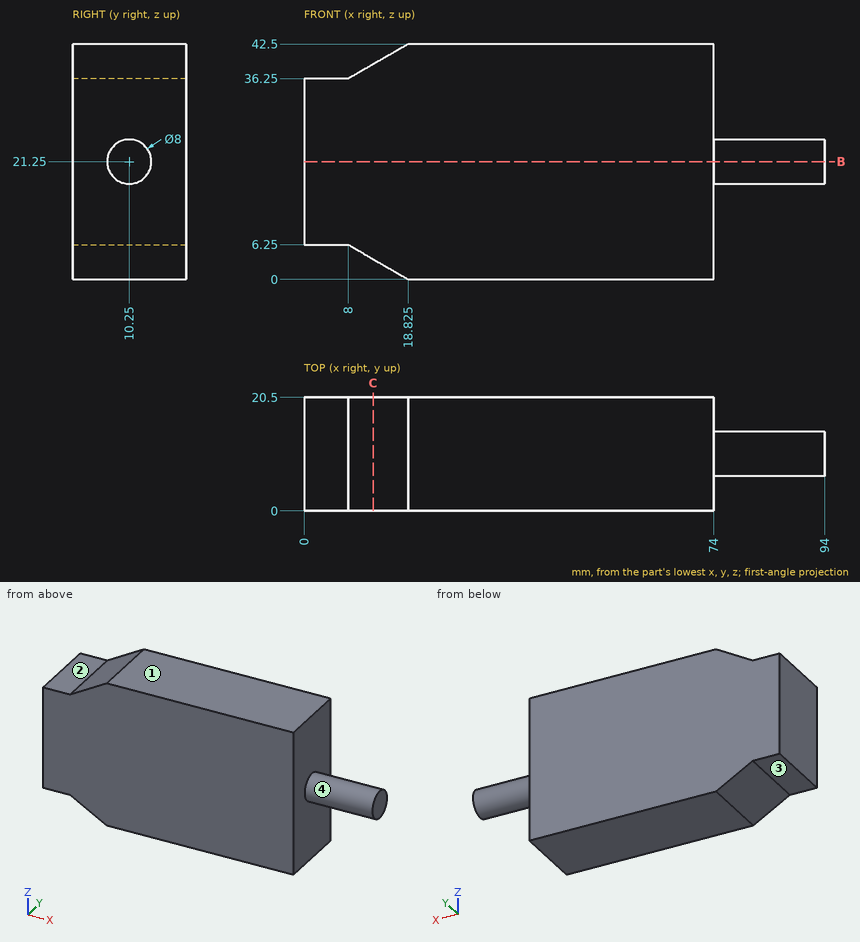
Input: dimensioned drawing with shaded views. Units: mm. Origin: part minimum x, y, z. A direction names the side the tool comes from. Coordinates: 2 decimals unless noted, no trailing zeros. Loops run counter-clockwise (first coordinate to the right, second up) from the corner with the lowest first, then second, coordinate; pieces in that order, holes last. Notation, with made-up numbers: (32, 2) -> (83, 2) arc R28 ccw to (83, 33) -> close; hole circle Ø9 at (16, 66). An arc over 180 degrees is marked (long way). Use a Markdown table: item, result. Add a question column.
(1) Access query for the marked faces 1, 2, 3 and 4. Directions: +Z, -Z, +X, -X, +Y, -Y. A direction counts if a zero-diameter tool reaches every point of the face in a straight line with its end or side. Return the directions, or none.
(2) Pin query (flat end, axial travel): pin 1 Ø2.5 at (x, y) = (3, 15) entering from -Z; pin 2 Ø4 at (x, y) = (2.5, 7.5) entering from +Z; pin 3 Ø3 at (y, z) = (3.5, 19.5) entering from +X. Return the tip coordinate at first contact, or that it passes through.
(3) Section query B-B, the plane z = 21.25. Return loops of the section in (x, y).
(4) Section query C-C, the plane x = 12.5. Return loops of the section in (y, z).
(5) Line query: line 1 along X through (y, z) = (9.25, 13); line 2 along Z through (x, y) = (7, 5); line 3 along X through (y, z) = (15.5, 3.5) (1 decimal). Output: solid intervals per line, ascending.
Answer:
| question | item | result |
|---|---|---|
| 1 | face 1 | +Z, +X, -X, +Y, -Y |
| 1 | face 2 | +Z, -X, +Y, -Y |
| 1 | face 3 | -Z, -X, +Y, -Y |
| 1 | face 4 | +X |
| 2 | pin 1 | stops at z = 6.25 |
| 2 | pin 2 | stops at z = 36.25 |
| 2 | pin 3 | stops at x = 74 |
| 3 | outline | (0, 0) -> (74, 0) -> (74, 6.25) -> (94, 6.25) -> (94, 14.25) -> (74, 14.25) -> (74, 20.5) -> (0, 20.5) -> close |
| 4 | outline | (0, 3.65) -> (20.5, 3.65) -> (20.5, 38.85) -> (0, 38.85) -> close |
| 5 | line 1 | x = 0 to 74 |
| 5 | line 2 | z = 6.25 to 36.25 |
| 5 | line 3 | x = 12.8 to 74 |
